The model under review builds one solid part; all positions refer to its coordinate system, in mm. Face numbers are marked on the shaded views. Round coordinates to 2 decimals unless told otherwise and drop trailing zeros. Order: outer loops, then holes, each group sorted by start corner. A loop starts at its lowest first (then second) coordinate and runs counter-clockwise, first axis right, second up. Notation, with made-up numbers: M -26,60.5 L -10,60.5 A4 ccw -10,65.5 Z; hole C -14.5,1 d9. An arc over 180 degrees is marked long. One line per item, written item: value. Start each with the question number.
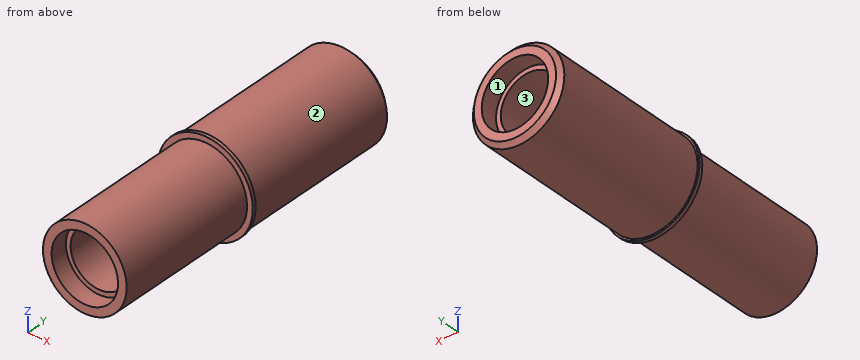
from build123d import *

# Parameters (mm, degrees)
CHAMFER1_SIZE = 1.524


with BuildPart() as part:
    # Sketch1 → Revolve1 (revolve)
    with BuildSketch(Plane(origin=(0, 0, 0), x_dir=(0, 0, -1), z_dir=(1, 0, 0)), mode=Mode.PRIVATE) as revolve1_sk:
        Polygon((11.09345, -53.086), (11.09345, -47.244), (9.525, -47.244), (9.525, 47.244), (11.09345, 47.244), (11.09345, 53.086), (15.2527, 53.086), (15.2527, -2.794000024), (15.875, -2.794000024), (15.875, -3.961), (13.97, -3.961), (13.97, -53.086), align=None)
    revolve(revolve1_sk.sketch.rotate(Axis((0, 53.086, 0), (0, -1, 0)), 180), axis=Axis((0, 53.086, 0), (0, -1, 0)))

    # Chamfer1
    chamfer1_edges = [part.edges().sort_by_distance(p)[0] for p in [
        (0, 53.086, -15.2527),
    ]]
    chamfer(chamfer1_edges, length=CHAMFER1_SIZE)


solid = part.part
Item 1: Consider section B-B, the plane y = -10. Give the boundary of the cut face in (x, z) (3 decimals).
Item 2: The part is to be moulded in two halves that separate along Z. For the marked faces 1, 2 and 3, say which applies: pulls with the +Z half, pulls with the -Z half, needs draft (parallel to the pull), parting line crosses it, or undercut.
Item 3: Consider section A-A, the plane z = 0. Give the boundary of the cut face in (x, y) (3 decimals).
Item 4: Wall thickness on L1, parallel to X at y = -51.5, z = 0; L2, parallel to X at y = -23, z = 0 (3 decimals); L3, parallel to Z at x = 7.5, y = 1: over which ranges is each line inside the solid? List them lowest first.
Item 5: Clearance check with flat-ended pins moving along their axes: P1, Ø10, axis at y = -6, z = 10, coming from the +X side; P2, Ø8, axis at x = 7, y = 21, coming from the -Z side; P3, Ø8, axis at y = 10.5, z = 12.5, coming from the -X side; P4, Ø11.5, axis at x = 0, z = 0, coming from the +Y side. State where each tip first meets the part, or that it passes through.
Computed:
1. outline: C 0,0 d27.94; hole C 0,0 d19.05
2. face 1: undercut
2. face 2: parting line crosses it
2. face 3: undercut
3. outline: M -15.875,-3.961 L -13.97,-3.961 L -13.97,-53.086 L -11.093,-53.086 L -11.093,-47.244 L -9.525,-47.244 L -9.525,47.244 L -11.093,47.244 L -11.093,53.086 L -13.729,53.086 L -15.253,51.562 L -15.253,-2.794 L -15.875,-2.794 Z; M 9.525,-47.244 L 11.093,-47.244 L 11.093,-53.086 L 13.97,-53.086 L 13.97,-3.961 L 15.875,-3.961 L 15.875,-2.794 L 15.253,-2.794 L 15.253,51.562 L 13.729,53.086 L 11.093,53.086 L 11.093,47.244 L 9.525,47.244 Z
4. L1: x = -13.97 to -11.09, 11.09 to 13.97
4. L2: x = -13.97 to -9.525, 9.525 to 13.97
4. L3: z = -13.28 to -5.87, 5.87 to 13.28
5. P1: stops at x = 14.92
5. P2: stops at z = -14.95
5. P3: stops at x = -12.66
5. P4: passes through
